Study the drawing (mm; zero at the part's minimum x, y, z) and answer. A direction names the side the tool comes from. Give positions to 0.01 mm unless a question says otherwise; leave off trailing zeros. Loops run counter-clockwise (first coordinate to the right, second up) from the corner with the lowest first, then second, coordinate; pieces in that order, holes last. Notation, with made-up numbers: (81.25, 29.5) - (103.25, 29.5) arc R28 cw to (103.25, 67.5) - close; hole circle Ø5 at (-0.75, 6). An arc over 180 degrees is marked (long way). Use one line per item in the form item = value. Start each with the question number.
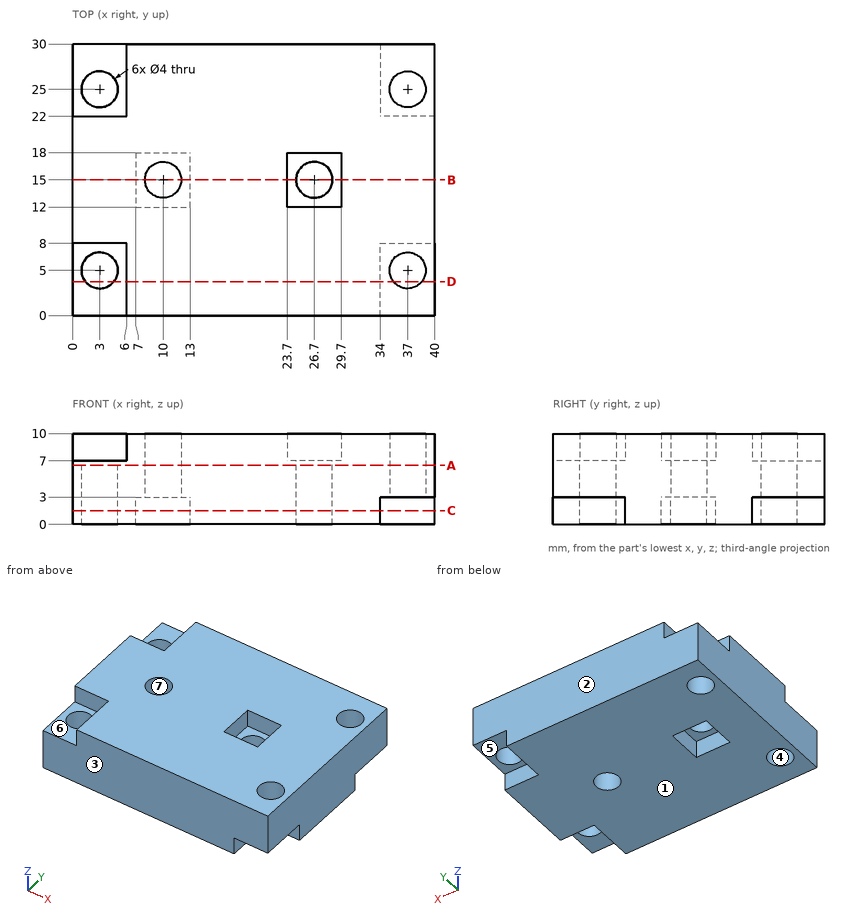
1) A cutting plane is placed at D-D (y = 3.75). Give the vertices of the cut face in (x, z).
2) Find the intervals of material crossed by probe 1 along Y at (x, z) = (3, 2); probe 2 along X at (y, z) = (13.75, 5.25); probe 3 along Y at (x, z) = (10, 1.75), in increasing order.
3) A tool of negligible diameter and unlimited length cuts with its end or side. For the marked faces 5, 6 and 7, from which of +Z, -Z, +X, -X, +Y, -Y can it reach the whole face along a straight path? Write none if from no direction.
4) Flat-ended cylindrical pins translate along their axes: pin 1 Ø0.9 at (y, z) = (4, 8) entering from -X; pin 2 Ø2 at (x, z) = (6.5, 3.5) entering from -Y; pin 3 Ø1.8 at (x, y) = (4, 28) entering from +Z; pin 4 Ø0.9 at (x, z) = (2.5, 9) entering from -Y. Find the tip coordinate at first contact, or state that the pin passes through.
5) A cutting plane is placed at A-A (z = 6.5). Give the vertices of the cut face in (x, y).
6) A cutting plane is placed at B-B (y = 15). Give the vertices of the cut face in (x, z).
7) A cutting plane is placed at C-C (z = 1.5). Give the vertices of the cut face in (x, y).
8) Determine the mould class of the marked faces 1, 2, 3 and 4 for opening direction Y: released by +Y, released by -Y, zero draft, split by the parting line, or undercut.
Answer sheet:
q1.outline = (0, 0) - (1.44, 0) - (1.44, 7) - (0, 7) - close; (4.56, 0) - (34, 0) - (34, 3) - (35.44, 3) - (35.44, 10) - (6, 10) - (6, 7) - (4.56, 7) - close; (38.56, 3) - (40, 3) - (40, 10) - (38.56, 10) - close
q2.probe_1 = 0 to 3, 7 to 23, 27 to 30
q2.probe_2 = 0 to 8.44, 11.56 to 25.14, 28.26 to 40
q2.probe_3 = 0 to 12, 18 to 30
q3.face_5 = -Z, +X, +Y
q3.face_6 = +Z, -X, -Y
q3.face_7 = +Z, -Z
q4.pin_1 = 6
q4.pin_2 = 0
q4.pin_3 = 7
q4.pin_4 = 8
q5.outline = (0, 0) - (40, 0) - (40, 30) - (0, 30) - close; hole circle Ø4 at (3, 5); hole circle Ø4 at (3, 25); hole circle Ø4 at (10, 15); hole circle Ø4 at (26.7, 15); hole circle Ø4 at (37, 5); hole circle Ø4 at (37, 25)
q6.outline = (0, 0) - (7, 0) - (7, 3) - (8, 3) - (8, 10) - (0, 10) - close; (12, 3) - (13, 3) - (13, 0) - (24.7, 0) - (24.7, 7) - (23.7, 7) - (23.7, 10) - (12, 10) - close; (28.7, 0) - (40, 0) - (40, 10) - (29.7, 10) - (29.7, 7) - (28.7, 7) - close
q7.outline = (0, 0) - (34, 0) - (34, 8) - (40, 8) - (40, 22) - (34, 22) - (34, 30) - (0, 30) - close; hole circle Ø4 at (3, 5); hole circle Ø4 at (3, 25); hole (7, 12) - (13, 12) - (13, 18) - (7, 18) - close; hole circle Ø4 at (26.7, 15)
q8.face_1 = zero draft
q8.face_2 = released by +Y
q8.face_3 = released by -Y
q8.face_4 = undercut
